Answer from the drawing. Dimensions are ordinates in mm from the lowest x, y and z of the part. A direction names the side the tool comes from. Coordinates: 2 decimals unless noted, no trailing zeros. Loops run counter-clockwise (first coordinate to the right, second up) from the corner with the lowest first, then second, coordinate; pieces in that order, holes last. Notation, with made-up numbers: M 47,0 L 105,0 A22 ccw 105,11 Z; hole C 3,34 d4. An arc over 180 degrees is marked long. Put each result on its own line as item: value.
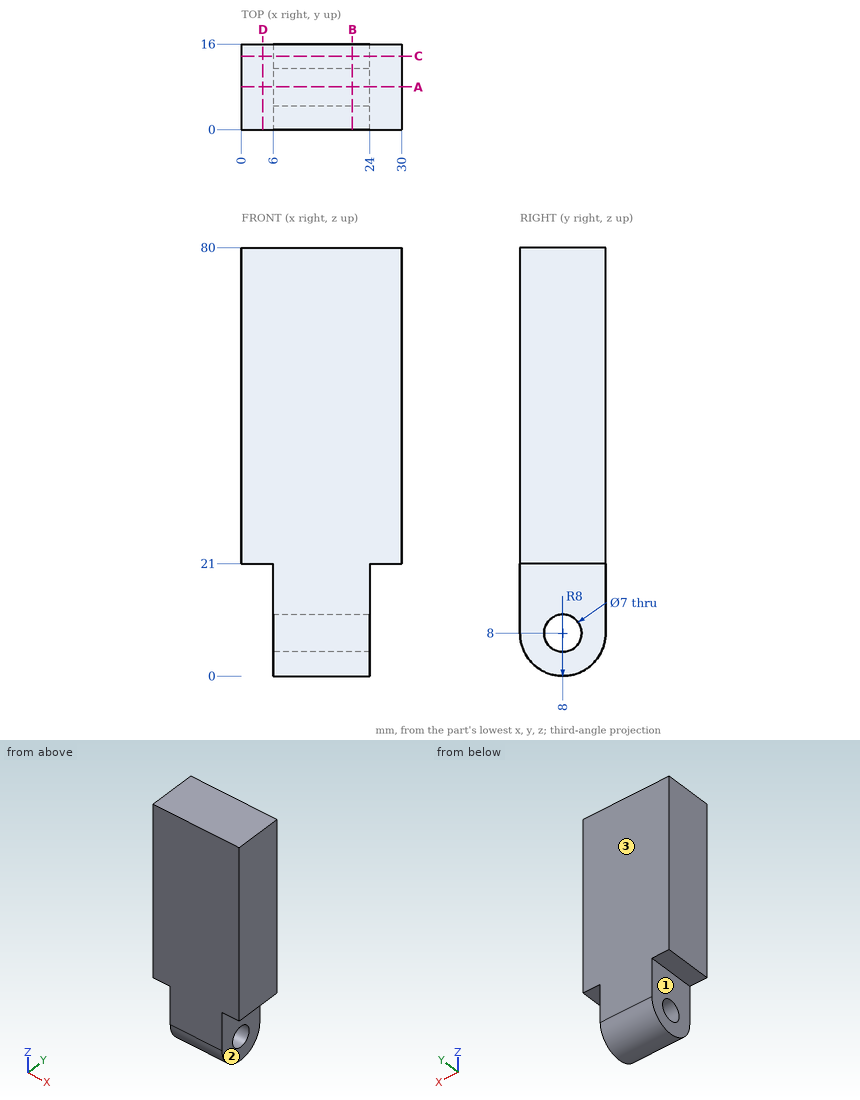
1) Find section D-D, the plane x = 4. Write down the section's boundary in (y, z).
Answer list:
outline: M 0,21 L 16,21 L 16,80 L 0,80 Z
2) Find section A-A, the plane y = 8. Write down the section's boundary in (x, z).
Answer list:
outline: M 0,21 L 6,21 L 6,11.5 L 24,11.5 L 24,21 L 30,21 L 30,80 L 0,80 Z; M 6,0 L 24,0 L 24,4.5 L 6,4.5 Z
3) Which of the six approach directions +Z, -Z, +X, -X, +Y, -Y give full straight-line access (tool end or side, diameter ignored) to the marked faces 1, 2 and 3?
Answer list:
face 1: -Z, -X, +Y, -Y
face 2: -Z, +X, +Y, -Y
face 3: +Z, -Z, +X, -X, +Y
4) Given pin 1 Ø8 at (y, z) = (8, 8) entering from -X; pin 2 Ø1.8 at (x, y) = (27, 6) entering from -Z; pin 3 Ø4 at (x, y) = (22, 12) entering from -Z, each flat-ended and moving along its own axis, determine where each tip first touches the part or whether it passes through.
Answer list:
pin 1: stops at x = 6
pin 2: stops at z = 21
pin 3: stops at z = 0.25
5) Straight lines are drawn through the part: line 1 (Y direction, x = 15.5, z = 8); line 2 (Z direction, x = 16, y = 8); line 3 (X direction, y = 2.5, z = 13). For each, find the intervals that lie inside material, in ascending order. Write a range as [from, to].
Answer list:
line 1: y = [0, 4.5], [11.5, 16]
line 2: z = [0, 4.5], [11.5, 80]
line 3: x = [6, 24]
6) Find section B-B, the plane x = 20.75. Write down the section's boundary in (y, z), plus the area to 3 significant figures.
Answer list:
outline: M 0,8 A8 ccw 16,8 L 16,80 L 0,80 Z; hole C 8,8 d7
area: 1,210 mm^2
7) Find section C-C, the plane y = 13.75. Write down the section's boundary in (x, z), plus the area to 3 significant figures.
Answer list:
outline: M 0,21 L 6,21 L 6,2.44 L 24,2.44 L 24,21 L 30,21 L 30,80 L 0,80 Z
area: 2,100 mm^2
